Geometry check sheet. Reference: the model listing, model coordinates, mm. A direction names the side the tool comes from. Coordinates: 2 decimals unless noted, no trailing zeros. Order: outer loops, then holes, each group sorted by start corner. A loop starts at its lowest first (then second) coordinate and runs counter-clockwise, first axis right, second up. Notation, with made-up numbers: (87, -36.75) - (131, -36.75) arc R12 ccw to (131, -15.75) - close; hole circle Ø10 at (19, -17). An arc over 180 degrees is marked (long way). Return JSON: item names as keys, results as strings. Group by question number.
Item 1: Section check A-A on y = 6.25. Enter the section's corners in (x, z), then the cut area to 3 significant figures.
Item 2: Section check B-B on x = -50.5. Enter the section's corners in (y, z).
Item 3: Scan lines: probe 1 along X at (y, z) = (6.25, 20); probe 2 along Z at (x, y) = (-104.5, 2.25); probe 3 along X at (y, z) = (6.25, 22). Record each from-to range of solid material in increasing order.
Item 4: Tool access check on faces 1 (the flat face through (-77.346, 6.162, 5.854)), 2 (the flat face through (-96, 6, 0)), 3 (the flat face through (-107, 0, 5)). Record the directions out of +Z, -Z, +X, -X, +Y, -Y that give a thin tool (end or side, any length) a straight path to the whole face; none if there is none.
Item 5: Gauge pin test, flat ends, axial feed: pin 1 (3 mm diameter, centred on x = -93.5, y = 2, fed in from +Z); pin 2 (4.5 mm diameter, centred on y = 3, z = 7.5, fed in from +X); pin 3 (2 mm diameter, centred on x = -148.5, y = 9.5, fed in from +Z). Record the tip position at first contact, or that the pin passes through.
Item 6: Section check C-C on x = -158. Enter the section's corners in (y, z).
Item 7: Draft check along X on faces 4 (the flat face through (-55.84, 6.16, 13.97)), 5 (the cylindrical face through (-153.61, 6.16, -8.35)), 6 (the flat face through (-167.027, 3.385, 8.931)), 7 (the flat face through (-37.9, 4.8, 26.776)). Enter one of: pulls with the +X half, pulls with the -X half, needs draft (parallel to the pull), parting line crosses it, or undercut.
from build123d import *

# Parameters (mm, degrees)
F0_W     = 13
F0_H     = 5.527861
F1_DEPTH = 12.5
F3_R     = 4.25
F4_DEPTH = 33.782
F2_R     = 4.25
F5_DEPTH = 25.4
F6_DEPTH = 25.4


with BuildPart() as f1:
    # F0 (on Front) → F1 (new body)
    with BuildSketch(Plane.XZ):
        with BuildLine():
            Line((-113.13897, 5.527861), (-113.13897, 11.055722))
            Line((-113.13897, 11.055722), (-121.63897, 11.055722))
            Line((-121.63897, 11.055722), (-149.829749, 0.795117))
            Line((-149.829749, 0.795117), (-164.829749, 26.77588))
            Line((-164.829749, 26.77588), (-177.329749, 26.77588))
            Line((-177.329749, 26.77588), (-160.275072, -2.763686))
            ThreePointArc((-160.275072, -2.763686), (-153.492043, -8.393653), (-144.678081, -8.251933))
            Line((-144.678081, -8.251933), (-145.446718, -8.550504))
            Line((-145.446718, -8.550504), (-121.954403, 0))
            Line((-121.954403, 0), (-113.13897, 0))
            Line((-113.13897, 0), (-113.13897, 5.527861))
        make_face()
        with Locations((-106.63897, 8.291791)):
            Rectangle(F0_W, F0_H)
        with Locations((-106.63897, 2.76393)):
            Rectangle(F0_W, F0_H)
        with BuildLine():
            Line((-53.119909, -2.966407), (-35.948191, 26.77588))
            Line((-35.948191, 26.77588), (-48.448191, 26.77588))
            Line((-48.448191, 26.77588), (-63.448191, 0.795117))
            Line((-63.448191, 0.795117), (-91.63897, 11.055722))
            Line((-91.63897, 11.055722), (-100.13897, 11.055722))
            Line((-100.13897, 11.055722), (-100.13897, 5.527861))
            Line((-100.13897, 5.527861), (-100.13897, 0))
            Line((-100.13897, 0), (-91.954403, 0))
            Line((-91.954403, 0), (-68.462087, -8.550504))
            ThreePointArc((-68.462087, -8.550504), (-59.774775, -8.550504), (-53.119909, -2.966407))
        make_face()
    extrude(amount=-F1_DEPTH)

    # F3 (on face) → F4 (cut)
    with BuildSketch(Plane.XY.offset(26.77588)):
        with Locations((-171.079749, 6.25)):
            Circle(F3_R)
    extrude(amount=-F4_DEPTH, mode=Mode.SUBTRACT)

    # F2 (on face) → F5 (cut)
    with BuildSketch(Plane.XY.offset(26.77588)):
        with Locations((-42.198191, 6.25)):
            Circle(F2_R)
    extrude(amount=-F5_DEPTH, mode=Mode.SUBTRACT)

    # F0 (on Front) → F6 (cut)
    with BuildSketch(Plane.XZ):
        with Locations((-106.63897, 8.291791)):
            Rectangle(F0_W, F0_H)
    extrude(amount=-F6_DEPTH, mode=Mode.SUBTRACT)


solid = f1.part
Computed:
{
 "1": {"outline": "(-177.33, 26.78) - (-175.33, 23.31) - (-175.33, 26.78) - close; (-166.83, 8.59) - (-160.28, -2.76) arc R12.7 ccw to (-144.68, -8.25) - (-145.45, -8.55) - (-121.95, 0) - (-91.95, 0) - (-68.46, -8.55) arc R12.7 ccw to (-53.12, -2.97) - (-46.45, 8.59) - (-46.45, 26.78) - (-48.45, 26.78) - (-63.45, 0.8) - (-91.64, 11.06) - (-100.14, 11.06) - (-100.14, 5.53) - (-113.14, 5.53) - (-113.14, 11.06) - (-121.64, 11.06) - (-149.83, 0.8) - (-164.83, 26.78) - (-166.83, 26.78) - close; (-37.95, 23.31) - (-35.95, 26.78) - (-37.95, 26.78) - close", "area": "1,520 mm²"},
 "2": {"outline": "(0, 1.57) - (12.5, 1.57) - (12.5, 23.22) - (0, 23.22) - close"},
 "3": {"probe 1": "x = -166.83 to -160.92, -52.36 to -46.45", "probe 2": "z = 0 to 5.53", "probe 3": "x = -166.83 to -162.07, -51.21 to -46.45"},
 "4": {"face 1": "+Z, +Y, -Y", "face 2": "-Z, +Y, -Y", "face 3": "+Z, -Z, +X, -X, -Y"},
 "5": {"pin 1": "stops at z = 11.06", "pin 2": "stops at x = -45.78", "pin 3": "stops at z = 1.64"},
 "6": {"outline": "(0, -5.64) - (12.5, -5.64) - (12.5, 14.95) - (0, 14.95) - close"},
 "7": {"face 4": "undercut", "face 5": "undercut", "face 6": "pulls with the -X half", "face 7": "needs draft"}
}
